```python
from build123d import *

# Parameters (mm, degrees)
F0_W = 6.3
F0_H = 10


with BuildPart() as f1:
    # F0 (on Front) → F1 (revolve)
    with BuildSketch(Plane.XZ):
        Polygon((0, 74), (0, 31.75), (7, 31.75), (7, 67), (33.3, 67), (33.3, 74), align=None)
        Polygon((33.3, 115.5), (33.3, 74), (33.3, 67), (38.8, 67), (38.8, 77), (38.8, 115.5), align=None)
        with Locations((41.95, 72)):
            Rectangle(F0_W, F0_H)
        Polygon((45.1, 77), (45.1, 67), (50.1, 67), (50.1, 115.5), (45.1, 115.5), align=None)
    revolve(axis=Axis((16.65, 0, 0), (1, 0, 0)))


solid = f1.part
```
Design review of the part built by this model. Coordinates are the model's own, in mm. A direction names the side the tool comes from. Coordinates: 2 decimals unless noted, no trailing zeros. Loops run counter-clockwise (first coordinate to the right, second up) from the corner with the lowest first, then second, coordinate; pieces in that order, holes last. Notation, with made-up numbers: (67, 43.5) - (80, 43.5) arc R19 ccw to (80, 51.5) - close; hole circle Ø5 at (60.5, 71). An arc over 180 degrees is marked (long way). Use CSV: the item, a comma, the result in double quotes. Start each with the question number.
1) Consider section D-D on y = -63. Write out the cut boundary in (x, z).
2) Wall thickness on L1, parallel to X at y = -30, z = 78; L2, parallel to Z at x = 29, y = 0; L3, parallel to Y at x = 34, z = 0: over which ranges is each line inside the solid? List them lowest first. Write a range as from..to.
3) Tool access review of faces 1 (the cylindrical face through (41.994, 46.853, -61.105)), 2 (the flat face through (7, 14, -29)), 3 (the cylindrical face through (36.012, 70.28, -91.657)), 4 (the cylindrical face through (16.42, 72.24, -16.04)), 5 (the flat face through (50.1, 50, -50)): name each direction out of +Z, -Z, +X, -X, +Y, -Y from which nothing blocks a thin tool from reaching the whole face with its end or side.
4) Consider section A-A on z = 0. Write out the cut boundary in (x, y), then the cut area to 3 significant figures.
5) Consider section C-C on x = 27. Write out the cut boundary in (y, z), then the cut area to 3 significant figures.
6) The part is to be moulded in two halves that separate along Y. For faces 6 (the cylindrical face through (28.852, 65.407, -14.524)), 7 (the cylindrical face through (47.565, 70.28, -91.657)), 8 (the flat face through (33.3, -2, 75)), say which applies: +Y half, -Y half, draft (parallel to the pull), parting line (faces both ways), or undercut.
7) For pin 1 Ø8 at (x, y) = (13.5, -58.5) entering from +Z; pin 2 Ø10 at (x, y) = (19, -29) entering from +Z; pin 3 Ø4 at (x, z) = (32, -41) entering from +Y, all flat-tipped, find the tip position at first contact; note any pin that passes through.
Geometry says:
1,outline,"(0, -38.82) - (33.3, -38.82) - (33.3, -96.81) - (38.8, -96.81) - (38.8, -44.27) - (45.1, -44.27) - (45.1, -96.81) - (50.1, -96.81) - (50.1, -22.8) - (7, -22.8) - (7, 22.8) - (50.1, 22.8) - (50.1, 96.81) - (45.1, 96.81) - (45.1, 44.27) - (38.8, 44.27) - (38.8, 96.81) - (33.3, 96.81) - (33.3, 38.82) - (0, 38.82) - close"
2,L1,"33.3..38.8, 45.1..50.1"
2,L2,"-74..-67, 67..74"
2,L3,"-115.5..-67, 67..115.5"
3,face 1,"none"
3,face 2,"+X"
3,face 3,"+X, -X"
3,face 4,"-X"
3,face 5,"+Z, -Z, +X, +Y, -Y"
4,outline,"(0, -74) - (33.3, -74) - (33.3, -115.5) - (38.8, -115.5) - (38.8, -77) - (45.1, -77) - (45.1, -115.5) - (50.1, -115.5) - (50.1, -67) - (7, -67) - (7, -31.75) - (0, -31.75) - close; (0, 31.75) - (7, 31.75) - (7, 67) - (50.1, 67) - (50.1, 115.5) - (45.1, 115.5) - (45.1, 77) - (38.8, 77) - (38.8, 115.5) - (33.3, 115.5) - (33.3, 74) - (0, 74) - close"
4,area,"2,100 mm^2"
5,outline,"circle Ø148 at (0, 0); hole circle Ø134 at (0, 0)"
5,area,"3,100 mm^2"
6,face 6,"undercut"
6,face 7,"parting line"
6,face 8,"draft"
7,pin 1,"z = 50.06"
7,pin 2,"z = 70"
7,pin 3,"y = 108.54"
